Part model, mm, in its own coordinate system. A direction names the side the tool comes from. Coordinates: 2 decimals unless noted, no trailing zeros. Write each loop counter-clockwise with the first axis right and the second up, starting at its lowest first coordinate (ties: lowest second). Pieces come first, ordered by that corner, then holes. Notation, with made-up numbers: (-3, -12) - (16, -12) arc R20 ccw to (16, 10) - close; hole circle Ø7 at (85.25, 58). An arc over 180 degrees is marked (long way). Use one line per item in the form item = value. Start each with the question number.
Autodesk Inventor part; units mm, degrees
ref_plane "YZ Plane" through (0, 0, 0) normal (1, 0, 0) x (0, 1, 0)
ref_plane "XZ Plane" through (0, 0, 0) normal (0, 1, 0) x (-1, 0, 0)
ref_plane "XY Plane" through (0, 0, 0) normal (0, 0, 1) x (1, 0, 0)
sketch "スケッチ1" plane through (0, 0, 0) normal (0, 1, 0) x (-1, 0, 0)
  line L0 (26, 0) -> (0, 0)
  line L1 (0, 0) -> (0, -30)
  line L2 (0, -30) -> (26, -30)
  line L3 (26, -30) -> (26, 0)
  line L4 (26, 0) -> (27.9445, -37.1034)
  line L5 (0, 0) -> (-1.9445, -37.1034)
  arc A0 (-1.9445, -37.1034) -> (27.9445, -37.1034) centre (13, 0) ccw
  line L6 (0, 0) -> (26, -30)
  line L7 (0, -30) -> (26, 0)
  line L8 (4, -4.6154) -> (22, -4.6154)
  line L9 (22, -4.6154) -> (22, -25.3846)
  line L10 (22, -25.3846) -> (4, -25.3846)
  line L11 (4, -25.3846) -> (4, -4.6154)
  circle A1 centre (4, -4.6154) radius 0.8
  circle A2 centre (4, -25.3846) radius 0.8
  circle A3 centre (22, -4.6154) radius 0.8
  circle A4 centre (22, -25.3846) radius 0.8
  dimension "d0" = 26
  dimension "d3" = 30
  dimension "d4" = 3
  dimension "d5" = 3
  dimension "d6" = 40
  dimension "d17" = 4
  dimension "d18" = 1.6
  dimension "d19" = 1.6
  dimension "d20" = 1.6
  dimension "d21" = 1.6
extrude "押し出し1" add sketch "スケッチ1" along normal blind 4 contours L7 A3 L8 A1 L6 L0 | L4 A0 L5 L1 L2 L3 | L3 L6 A4 L9 A3 L7 | L6 A1 L11 A2 L7 L1 | L2 L7 A2 L10 A4 L6 | A3 L7 L6 A1 L8 | A1 L6 L7 A2 L11 | L10 A2 L7 L6 A4 | A3 L9 A4 L6 L7
sketch "スケッチ2" plane through (0, 0, 0) normal (0, -1, 0) x (1, 0, 0)
  arc A0 (-25.871, -35.7538) -> (-0.129, -35.7538) centre (-13, 0) ccw
  arc A1 (-27.9445, -37.1034) -> (1.9445, -37.1034) centre (-13, 0) ccw
  line L0 (-0.129, -35.7538) -> (-0.6849, -25.1463)
  line L1 (-25.871, -35.7538) -> (-25.3151, -25.1463)
  arc A2 (-25.3151, -25.1463) -> (-0.6849, -25.1463) centre (-13, 0) ccw
  line L2 (0, 0) -> (1.9445, -37.1034)
  line L3 (-27.9445, -37.1034) -> (-26, 0)
  line L4 (-26, 0) -> (0, 0)
  circle A3 centre (-4, -4.6154) radius 0.8
  circle A4 centre (-22, -4.6154) radius 0.8
  circle A5 centre (-22, -25.3846) radius 0.8
  circle A6 centre (-4, -25.3846) radius 0.8
  dimension "d9" = 2
  dimension "d10" = 2
  dimension "d11" = 2
  dimension "d12" = 10
extrude "押し出し3" add sketch "スケッチ2" along normal blind 1
fillet "フィレット1" radius 0.5 4 edges at (-13, -1, -28) (-0.4069, -1, -30.4501) (-13, -1, -38) (-25.5931, -1, -30.4501)
fillet "フィレット2" radius 2 4 edges at (-27.9445, 1.5, -37.1034) (1.9445, 1.5, -37.1034) (0, 1.5, 0) (-26, 1.5, 0)
sketch "スケッチ3" plane through (0, -1, 0) normal (0, -1, 0) x (1, 0, 0)
  circle A0 centre (-4, -4.6154) radius 0.8
  circle A1 centre (-22, -4.6154) radius 0.8
  arc A2 (-21.6502, -26.1041) -> (-22.7249, -25.7231) centre (-22, -25.3846) ccw
  arc A3 (-3.2751, -25.7231) -> (-4.3498, -26.1041) centre (-4, -25.3846) ccw
  circle A4 centre (-4, -4.6154) radius 2
  circle A5 centre (-22, -4.6154) radius 2
  circle A6 centre (-22, -25.3846) radius 2
  circle A7 centre (-4, -25.3846) radius 2
  point P0 (0, 0)
  dimension "d22" = 4
  dimension "d23" = 4
  dimension "d24" = 4
  dimension "d25" = 4
extrude "押し出し4" cut sketch "スケッチ3" against normal blind 2 contours A0 | A1 | A4 | A5 | A6 | A7
properties part number "toe_sole_back"
Q1. Slice it at B-B (z = -8). List the corners of the cut face in (x, y).
Q2. Slice it at A-A (y = 3.4). List the corners of the cut face in (x, z).
Q3. Pin check, flat tips, straight feed: P1, Ø1.2, axis at x = -22, z = -25, coming from the -Y side; P2, Ø1.5, axis at x = -8, y = -0.5, coming from the -Z side; P3, Ø3, axis at y = 0, z = -10.5, coming from the +X side; P4, Ø1, axis at x = -4, z = -4.62, coming from the +Y side. Stop position of each tip, or through.
Q4. Which spindle directions (+Z, -Z, +X, -X, +Y, -Y) get a long thin tool onto all of the face, cutting with end or side? Do faces 1 (the cylindrical face through (-13, 2, -40)), 2 (the flat face through (-3, 1, -5)). Say none if no direction does.
Q5. Drill centre lines: probe 1 along Z at (x, y) = (-22, 0.2); probe 2 along Z at (x, y) = (-22, -0.55); probe 3 along Y at (x, z) = (-11.5, -29.5). Where is each one in solid material? Low to high.
Q6. Slice it at D-D (y = 0.55). List the corners of the cut face in (x, z), plus the area to 3 significant figures.
Q7. Slice it at C-C (x = -4). Count the separate pieces of the cut face and the enclosed holes in it, plus the area to 3 significant figures.
Solution:
q1.outline = (-26.42, -1) - (0.42, -1) - (0.42, 4) - (-26.42, 4) - close
q2.outline = (-27.87, -35.65) arc R2 ccw to (-26.55, -37.64) arc R40 ccw to (0.55, -37.64) arc R2 ccw to (1.87, -35.65) - (0.1, -1.9) arc R2 ccw to (-1.9, 0) - (-24.1, 0) arc R2 ccw to (-26.1, -1.9) - close; hole circle Ø1.6 at (-22, -25.38); hole circle Ø1.6 at (-22, -4.62); hole circle Ø1.6 at (-4, -25.38); hole circle Ø1.6 at (-4, -4.62)
q3.P1 = 1
q3.P2 = -39.77
q3.P3 = 0.63
q3.P4 = through
q4.face_1 = -Z, +Y, -Y
q4.face_2 = -Y
q5.probe_1 = -38.97 to -27.38, -23.38 to -6.62, -2.62 to 0
q5.probe_2 = -38.97 to -36.92, -23.38 to -6.62, -2.62 to 0
q5.probe_3 = 0 to 4
q6.outline = (-27.87, -35.65) arc R2 ccw to (-26.55, -37.64) arc R40 ccw to (0.55, -37.64) arc R2 ccw to (1.87, -35.65) - (0.1, -1.9) arc R2 ccw to (-1.9, 0) - (-24.1, 0) arc R2 ccw to (-26.1, -1.9) - close; hole circle Ø4 at (-22, -25.38); hole circle Ø4 at (-22, -4.62); hole circle Ø4 at (-4, -25.38); hole circle Ø4 at (-4, -4.62)
q6.area = 1,040 mm2
q7.separate_pieces = 3
q7.enclosed_holes = 0
q7.area = 160 mm2
